Read the model definition and answer for the solid it produces. Units are mm, in the model's axes. A direction names the side the tool comes from. Give positions to 0.01 mm unless a question says otherwise; leave off trailing zeros. Loops run counter-clockwise (first coordinate to the right, second up) from the corner with the lowest first, then second, coordinate; pieces in that order, holes last. Notation, with made-up numbers: (70, 42.25) - (109, 42.25) arc R19 cw to (109, 78.25) - close; hole circle Ø5 at (29.25, -3.5). An arc over 180 degrees is marked (long way). Use a Markdown table: item, result. Add a question column.
Item 1: A cutting plane is placed at B-B (x = 51). Determine the outline of the cut face in (y, z).
Item 2: Which of the six approach directions +Z, -Z, +X, -X, +Y, -Y give full straight-line access (tool end or side, diameter ignored) to faces 1 (the face through (79.72, 10.648, -13.887)), 2 (the face through (47.561, 13, 13)), 3 (the face through (-79.72, 10.648, -13.887)), 4 (the face through (-100, 0, 0)), 5 (the face through (100, 0, 0))?
Item 3: Consider probe 1 along X at (y, z) = (18, 19.5); probe 2 along Z at (x, y) = (-49, 23); probe 3 along Z at (x, y) = (69, 13). Determine where each line is inside the solid, lowest interval first. Write a range as [from, to].
Item 4: For a pull along X with two mould halves and no side action, classify faces 6 (the face through (53.69, -1.32, -29.97)), 7 (the face through (60, 13, -13)), 8 (the face through (-47.561, 13, 13)) as +X half, -X half, draft (parallel to the pull), parting line (faces both ways), or undercut.
Item 5: A cutting plane is placed at A-A (y = -24.5). Determine the outline of the cut face in (x, z), plus the area to 3 significant figures.
Item 6: This flat-tipped pin is pushed along its axis until it touches: P1, Ø5, axis at y = 7.5, z = 23, coming from the -X side. Where does it stop, or does it pass through?
from build123d import *


with BuildPart() as f1:
    # F0 (on Front) → F1 (revolve)
    with BuildSketch(Plane.XZ):
        with BuildLine():
            Line((47.5609842221, 30), (47.5609842221, 17.5))
            add(Edge.make_bspline(
                [(21.6804631054, 9.5182526857), (30.3073034776, 12.1788351238), (38.9341438499, 14.8394175619), (47.5609842221, 17.5)],
                knots=[0, 0, 0, 0, 27.0833835305, 27.0833835305, 27.0833835305, 27.0833835305], degree=3))
            add(Edge.make_bspline(
                [(21.6804631054, 9.5182526857), (14.4536420703, 9.2621684571), (7.2268210351, 9.0060842286), (0, 8.75)],
                knots=[0, 0, 0, 0, 21.6940704492, 21.6940704492, 21.6940704492, 21.6940704492], degree=3))
            Line((0, 8.75), (0, 0))
            Line((0, 0), (100, 0))
            Line((100, 0), (100, 17.5))
            Line((100, 17.5), (60, 17.5))
            Line((60, 17.5), (60, 30))
            Line((60, 30), (47.5609842221, 30))
        make_face()
    revolve(axis=Axis((50, 0, 0), (1, 0, 0)))

    # F2: F1 across face


with BuildPart() as f1_1:
    add(f1.part)
    add(f1.part.mirror(Plane(origin=(0, 0, 0), x_dir=(0, -1, 0), z_dir=(-1, 0, 0))))


solid = f1_1.part
Geometry says:
| question | item | result |
|---|---|---|
| 1 | outline | circle Ø60 at (0, 0) |
| 2 | face 1 | +X |
| 2 | face 2 | none |
| 2 | face 3 | -X |
| 2 | face 4 | +Z, -Z, -X, +Y, -Y |
| 2 | face 5 | +Z, -Z, +X, +Y, -Y |
| 3 | probe 1 | [-60, -47.56], [47.56, 60] |
| 3 | probe 2 | [-19.26, 19.26] |
| 3 | probe 3 | [-11.72, 11.72] |
| 4 | face 6 | draft |
| 4 | face 7 | +X half |
| 4 | face 8 | undercut |
| 5 | outline | (-60, -17.31) - (-47.56, -17.31) - (-47.56, 17.31) - (-60, 17.31) - close; (47.56, -17.31) - (60, -17.31) - (60, 17.31) - (47.56, 17.31) - close |
| 5 | area | 861 mm² |
| 6 | P1 | x = -60 |
